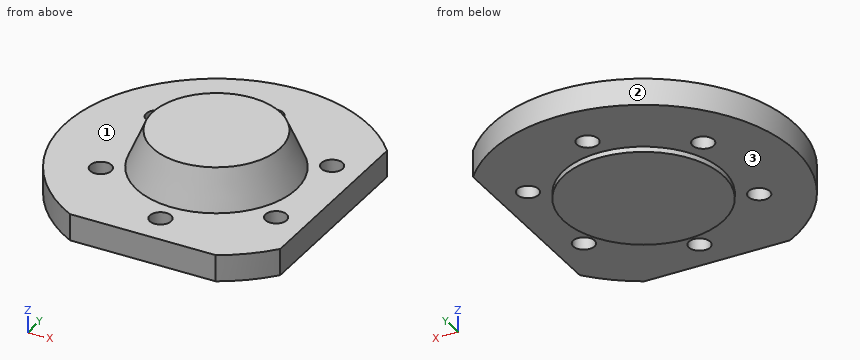
from build123d import *

# Parameters (mm, degrees)
SKETCH1_R           = 15
SKETCH1_R_2         = 2
BOSS_EXTRUDE1_DEPTH = 5
SKETCH1_2_R         = 15
BOSS_EXTRUDE2_DEPTH = 6
SKETCH2_R           = 12
SKETCH1_4_R         = 15


with BuildPart() as part:
    # Sketch1 → Boss-Extrude1 (new body)
    with BuildSketch(Plane.XY):
        with BuildLine():
            Line((22, -18.117670932), (22, 18.117670932))
            ThreePointArc((22, 18.117670932), (-21.956152501, 18.170783345), (-13.683932183, -25))
            Line((-13.683932183, -25), (13.683932183, -25))
            ThreePointArc((13.683932183, -25), (18.170783345, -21.956152501), (22, -18.117670932))
        make_face()
        Circle(SKETCH1_R, mode=Mode.SUBTRACT)
        with Locations((0, 19)):
            Circle(SKETCH1_R_2, mode=Mode.SUBTRACT)
        with Locations((16.454482672, 9.5)):
            Circle(SKETCH1_R_2, mode=Mode.SUBTRACT)
        with Locations((16.454482672, -9.5)):
            Circle(SKETCH1_R_2, mode=Mode.SUBTRACT)
        with Locations((0, -19)):
            Circle(SKETCH1_R_2, mode=Mode.SUBTRACT)
        with Locations((-16.454482672, -9.5)):
            Circle(SKETCH1_R_2, mode=Mode.SUBTRACT)
        with Locations((-16.454482672, 9.5)):
            Circle(SKETCH1_R_2, mode=Mode.SUBTRACT)
    extrude(amount=-BOSS_EXTRUDE1_DEPTH)

    # Sketch1<2> → Boss-Extrude2 (add)
    with BuildSketch(Plane.XY):
        Circle(SKETCH1_2_R)
    extrude(amount=-BOSS_EXTRUDE2_DEPTH)

    # Sketch2 → Loft1 section 0
    with BuildSketch(Plane.XY.offset(7)):
        Circle(SKETCH2_R)
    # Sketch1<4> → Loft1 section 1
    with BuildSketch(Plane.XY):
        Circle(SKETCH1_4_R)
    loft()


solid = part.part
The listing builds one solid part. Answer for the finished solid, in the listing's coordinates (mm). Face numbers are marked on the shaded views. A direction names the side the tool comes from. Give positions to 0.01 mm unless a question says otherwise; leave off trailing zeros. Order: outer loops, then holes, each group sorted by start corner. A loop starts at its lowest first (then second) coordinate and runs counter-clockwise, first axis right, second up. Notation, with made-up numbers: (42, 24) - (71, 24) arc R26 cw to (71, 40) - close; hole circle Ø3 at (-11.75, 28). An arc over 180 degrees is marked (long way). Answer as CSV lines item,"result".
Q1. Which of the six approach directions +Z, -Z, +X, -X, +Y, -Y give full straight-line access (tool end or side, diameter ignored) to the marked faces 1, 2 and 3?
Answer key:
face 1,"+Z"
face 2,"+Z, -Z"
face 3,"-Z"
Q2. A cutting plane is placed at B-B, the plane z = -2. Determine the outline of the cut face in (x, y), and give its area (3 significant figures).
Answer key:
outline,"(-13.68, -25) - (13.68, -25) arc R28.5 ccw to (22, -18.12) - (22, 18.12) arc R28.5 ccw (long way) to start; hole circle Ø4 at (-16.45, -9.5); hole circle Ø4 at (-16.45, 9.5); hole circle Ø4 at (0, -19); hole circle Ø4 at (0, 19); hole circle Ø4 at (16.45, -9.5); hole circle Ø4 at (16.45, 9.5)"
area,"2,250 mm^2"
Q3. A cutting plane is placed at C-C, the plane y = 19. Determine the outline of the cut face in (x, z), and give its area (3 significant figures).
Answer key:
outline,"(-21.24, -5) - (-2, -5) - (-2, 0) - (-21.24, 0) - close; (2, -5) - (21.24, -5) - (21.24, 0) - (2, 0) - close"
area,"192 mm^2"
Q4. Straight lines are drawn through the part: L1, parallel to Y at x = 0, z = -3.95; L2, parallel to Y at x = -17.5, z = -2.75; L3, parallel to Z at x = -1, y = 24. For each, find the intervals that lie inside material, in ascending order.
Answer key:
L1,"y = -25 to -21, -17 to 17, 21 to 28.5"
L2,"y = -22.49 to -11.2, -7.8 to 7.8, 11.2 to 22.49"
L3,"z = -5 to 0"
Q5. A cutting plane is placed at D-D, the plane y = -9.5. Count the separate pieces of the cut face and the enclosed holes in it, and give its area (3 significant figures).
Answer key:
separate pieces,"3"
enclosed holes,"0"
area,"361 mm^2"
Q6. Each of these flat-tipped pins is pushed along its axis until it touches: pin 1 Ø5 at (x, y) = (-16.45, -9.5) entering from -Z; pin 2 Ø3 at (x, y) = (16.45, 9.5) entering from +Z; pin 3 Ø2 at (x, z) = (-11.5, 2.5) entering from +Y; pin 4 Ø5 at (x, z) = (-20, 0) entering from +Y. Where does it stop, or does it pass through?
Answer key:
pin 1,"stops at z = -5"
pin 2,"passes through"
pin 3,"stops at y = 9.32"
pin 4,"stops at y = 22.49"
Q7. A cutting plane is placed at A-A, the plane x = 0. Determine the outline of the cut face in (y, z), and give its area (4 significant figures).
Answer key:
outline,"(-25, -5) - (-21, -5) - (-21, 0) - (-25, 0) - close; (-17, -5) - (-15, -5) - (-15, -6) - (15, -6) - (15, -5) - (17, -5) - (17, 0) - (15, 0) - (12, 7) - (-12, 7) - (-15, 0) - (-17, 0) - close; (21, -5) - (28.5, -5) - (28.5, 0) - (21, 0) - close"
area,"446.5 mm^2"
